The figure shows three views and two pictorial views of one solid part (mm, origin at its lowest corner). Answer the questions. A direction names the side the tool comes from. Coordinates: 2 decimals unless noted, no trailing zeros. Order: outer loops, then holes, each group sorted by start corner. A loop starts at its lowest first (then second) coordinate and runs counter-clockwise, first axis right, second up. Notation, with made-up numbers: (32, 61.25) - (66, 61.25) arc R16 cw to (66, 71.25) - close; hole circle Ø5 at (71.25, -37.5). An arc over 180 degrees is marked (long way). Use one line per item in the form item = value.
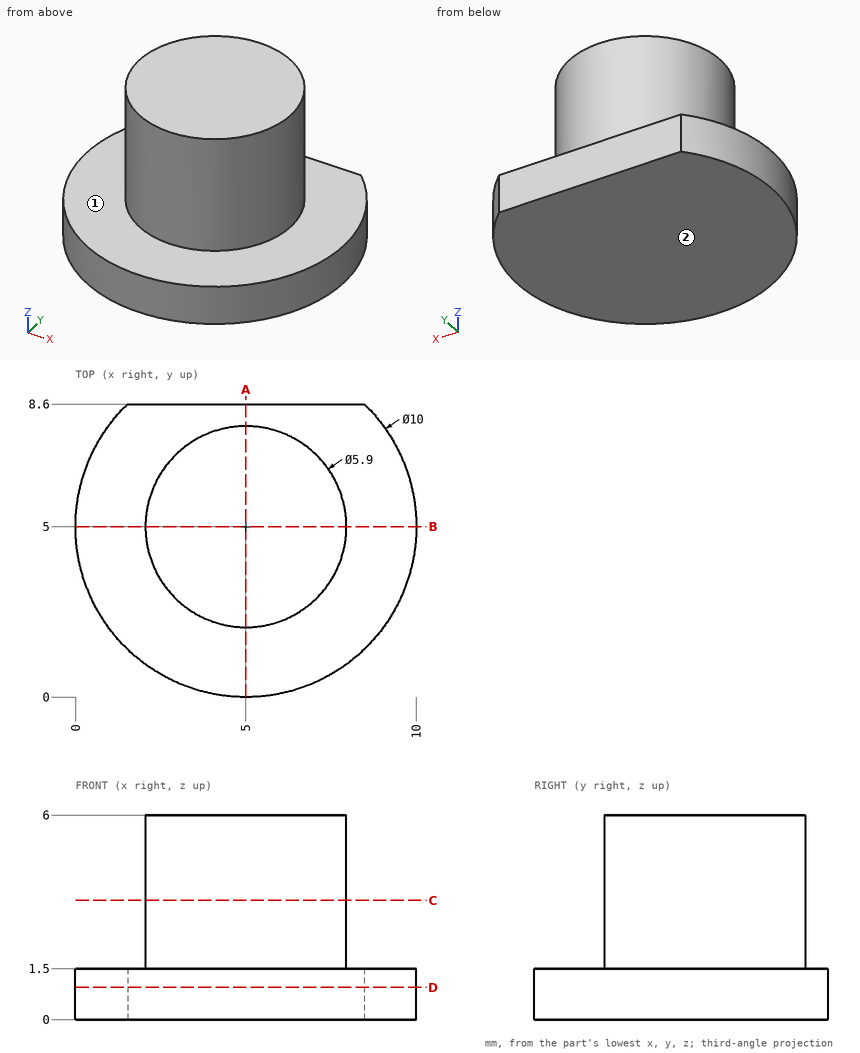
(1) Straight lines are drawn through the part: L1, parallel to Z at x = 7.75, y = 8; L2, parallel to X at y = 7.5, z = 2.95; L3, parallel to X at y = 3.5, z = 4.6. For each, find the intervals that lie inside material, in ascending order.
Answer list:
L1 = 0 to 1.5
L2 = 3.43 to 6.57
L3 = 2.46 to 7.54
(2) Section C-C, the plane z = 3.5 is taken. Write down the section's boundary in (x, y), then the cut area to 3 significant figures.
Answer list:
outline = circle Ø5.9 at (5, 5)
area = 27.3 mm2
(3) Section B-B, the plane y = 5 is taken. Write down the section's boundary in (x, z).
Answer list:
outline = (0, 0) - (10, 0) - (10, 1.5) - (7.95, 1.5) - (7.95, 6) - (2.05, 6) - (2.05, 1.5) - (0, 1.5) - close
(4) Section A-A, the plane x = 5 is taken. Write down the section's boundary in (y, z), then the cut area to 4 significant figures.
Answer list:
outline = (0, 0) - (8.6, 0) - (8.6, 1.5) - (7.95, 1.5) - (7.95, 6) - (2.05, 6) - (2.05, 1.5) - (0, 1.5) - close
area = 39.45 mm2
(5) Section D-D, the plane z = 0.95 is taken. Write down the section's boundary in (x, y), then the cut area to 3 significant figures.
Answer list:
outline = (1.53, 8.6) arc R5 ccw (long way) to (8.47, 8.6) - close
area = 71.9 mm2
(6) Given pin 1 Ø1 at (x, y) = (8.5, 3.5) entering from +Z, flat-ended and moving along its own axis, determine where the tip first touches the part or whether it passes through.
Answer list:
pin_1 = 1.5
(7) Which of the six approach directions +Z, -Z, +X, -X, +Y, -Y give full straight-line access (tool end or side, diameter ignored) to the marked faces 1 and 2?
Answer list:
face_1 = +Z
face_2 = -Z, +X, -X, +Y, -Y
